```python
from build123d import *

# Parameters (mm, degrees)
ESQUISSE1_R             = 55
ESQUISSE1_R_2           = 25
BOSS_EXTRU_1_DEPTH      = 6
BOSS_EXTRU_2_DEPTH      = 1
BOSS_EXTRU_2_DEPTH_BACK = 6
ESQUISSE2_R             = 25
ESQUISSE2_R_2           = 21
ESQUISSE4_R             = 25
ESQUISSE4_R_2           = 21
ESQUISSE8_R             = 25
ESQUISSE8_R_2           = 23.5
ENL_V_MAT_EXTRU_1_DEPTH = 38


with BuildPart() as part:
    # Esquisse1 → Boss.-Extru.1 (new body)
    with BuildSketch(Plane.XY):
        Circle(ESQUISSE1_R)
        Circle(ESQUISSE1_R_2, mode=Mode.SUBTRACT)
    extrude(amount=BOSS_EXTRU_1_DEPTH)

    # Esquisse2 → Boss.-Extru.2 (add, two sides: drawn at the far end of the back side and taken through both)
    with BuildSketch(Plane.XY.offset(6).offset(-BOSS_EXTRU_2_DEPTH_BACK)):
        Circle(ESQUISSE2_R)
        Circle(ESQUISSE2_R_2, mode=Mode.SUBTRACT)
    extrude(amount=BOSS_EXTRU_2_DEPTH + BOSS_EXTRU_2_DEPTH_BACK)

    # Balayage5: sweep along a path in Esquisse3
    with BuildLine(Plane(origin=(0, 0, 0), x_dir=(0, 0, -1), z_dir=(1, 0, 0))) as balayage5_path:
        Line((-7, 0), (-17, 0))
        ThreePointArc((-17, 0), (-42.711504387, 9.358222275), (-56.39231012, 33.054072893))
        Line((-56.39231012, 33.054072893), (-63.338237227, 72.446383014))
    # Esquisse4 → Balayage5 (sweep)
    with BuildSketch(Plane.XY.offset(7)):
        Circle(ESQUISSE4_R)
        Circle(ESQUISSE4_R_2, mode=Mode.SUBTRACT)
    sweep(path=balayage5_path.line)

    # Esquisse8 → Enlèv. mat.-Extru.1 (cut)
    with BuildSketch(Plane(origin=(0, 81.093333754, 14.298942697), x_dir=(1, 0, 0), z_dir=(0, 0.9848077530122087, 0.17364817766692714))):
        with Locations(Location((0, -49.795804695, 0), (0, 0, 270))):
            Circle(ESQUISSE8_R)
        with Locations(Location((0, -49.795804695, 0), (0, 0, 270))):
            Circle(ESQUISSE8_R_2, mode=Mode.SUBTRACT)
    extrude(amount=-ENL_V_MAT_EXTRU_1_DEPTH, mode=Mode.SUBTRACT)


solid = part.part
```
CAD build for the part. Positions are in the model's coordinates, mm. A direction names the side the tool comes from. Round coordinates to 2 decimals unless told otherwise and drop trailing zeros. Write each loop counter-clockwise with the first axis right and the second up, starting at its lowest first coordinate (ties: lowest second). Pieces come first, ordered by that corner, then holes.
Item 1: Mould opens along X. For faces 1 (the cylindrical face through (23.846, 35.357, 49.173)), 2 (the flat face through (-9.143, 31.185, 78.509)), 3 (the cylindrical face through (20.03, 54.12, 53.7)), 4 (the cylindrical face through (20.03, 6.31, 8.38)) say: released by +X, released by -X, zero draft, split by the parting line, or undercut.
Filled in:
face 1: split by the parting line
face 2: zero draft
face 3: undercut
face 4: undercut
Item 2: Band-saw the part on A-A on x = 0. Write the cut outline in (y, z).
Filled in:
outline: (-55, 0) - (-21, 0) - (-21, 17) arc R61 cw to (29.41, 77.07) - (68.8, 84.02) - (68.37, 86.48) - (30.94, 79.88) - (30.68, 81.36) - (28.71, 81.01) arc R65 ccw to (-25, 17) - (-25, 6) - (-55, 6) - close; (21, 0) - (55, 0) - (55, 6) - (25, 6) - (25, 17) arc R15 cw to (37.4, 31.77) - (39.36, 32.12) - (39.1, 33.6) - (76.53, 40.2) - (76.09, 42.66) - (36.7, 35.71) arc R19 ccw to (21, 17) - close
Item 3: Band-saw the part on C-C on x = -40.5. Write the cut outline in (y, z), then the cut area to 3 significant figures.
Filled in:
outline: (-37.21, 0) - (37.21, 0) - (37.21, 6) - (-37.21, 6) - close
area: 447 mm2
Item 4: Tool access for faces 5 (the flat face through (-1, -24, 0)), 6 (the flat face through (11, -24, 6)): list every direction of +Z, -Z, +X, -X, +Y, -Y with a clear straight run to the whole face (end or side of a thin tool).
Filled in:
face 5: -Z, +X, -X, +Y, -Y
face 6: none
Item 5: Band-saw the part on B-B on y = 51.5. Give the number of separate pieces and of enclosed holes in the cut face, then the cut area to 3 significant figures.
Filled in:
separate pieces: 2
enclosed holes: 1
area: 587 mm2
Item 6: Drop flat-ended pins along their axis: pin 1 Ø25 at (x, y) = (0, 0) entering from +Z; pin 2 Ø2 at (x, y) = (15.5, 15) entering from -Z; pin 3 Ø1.5 at (x, z) = (-13, 65) entering from -Y; pin 4 Ø1 at (x, y) = (37, 26.5) entering from +Z. Give the stop position or say it passes through.
Filled in:
pin 1: stops at z = 75.9
pin 2: stops at z = 0
pin 3: stops at y = 0.62
pin 4: stops at z = 6
Item 7: Drill centre lines: L1, parallel to Y at x = 0, z = 9; L2, parallel to Y at x = 0, z = 4.75. Where is each one in solid material? Low to high.
Filled in:
L1: y = -25 to -21, 21 to 25
L2: y = -55 to -21, 21 to 55
